Verification items for the finished model (mm, model axes). Face numbers are marked on the shaded views. A direction names the side the tool comes from. Round coordinates to 2 decimals unless told otherwise and drop trailing zeros. Order: outer loops, then holes, each group sorted by start corner. A loop starts at its lowest first (then second) coordinate and runs counter-clockwise, first axis right, second up. Notation, with made-up numbers: (67.5, 0) -> (97.5, 0) arc R11 ccw to (97.5, 4) -> close; hole circle Ø8 at (-30.75, 21.5). An arc over 180 degrees is marked (long way). Return JSON: item names as keys, results as strings. Group by question number.
Item 1: Depth check by flat-ended pin: pin 1 Ø2 at (y, z) = (-27, 3.5) entering from -X; pin 2 Ø1.6 at (x, z) = (-4.5, 3) entering from +Y; pin 3 Ø5 at (x, y) = (6, -23.5) entering from +Z. Enter the tip coordinate at first touch or a pass-through.
Item 2: Scan lines: probe 1 along X at (y, z) = (-23, 0.7); probe 2 along Z at (x, y) = (1.5, -26.5); probe 3 along X at (y, z) = (-24.75, 2.25). Record each from-to range of solid material in increasing order. Write a range as from..to.
Item 3: Sectioned sample at D-D on x = 7.5. Record the cut outline in (y, z).
Item 4: Sectioned sample at C-C on z = 2.5. Record the cut outline in (x, y).
Item 5: Access from +Z, -Z, +X, -X, +Y, -Y to the whole of each face (thin tool, end or side, straight path). Record for the marked faces 1, 2 and 3.
Item 6: Sectioned sample at A-A on y = -26. Record the cut outline in (x, z), plus the area to 3 significant figures.
Item 7: Sectioned sample at B-B on x = -4.25. Record the cut outline in (y, z), plus the area to 3 significant figures.
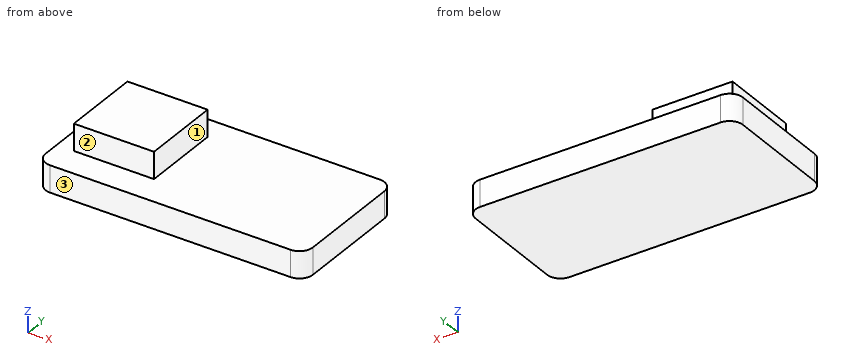
```python
from build123d import *

# Parameters (mm, degrees)
SKETCH1_W           = 20
SKETCH1_H           = 10
BOSS_EXTRUDE1_DEPTH = 2
FILLET1_R           = 1
SKETCH2_W           = 6
SKETCH2_H           = 6
BOSS_EXTRUDE2_DEPTH = 2


with BuildPart() as part:
    # Sketch1 → Boss-Extrude1 (new body)
    with BuildSketch(Plane.XY):
        with Locations((0, -27.096458497)):
            Rectangle(SKETCH1_W, SKETCH1_H)
    extrude(amount=BOSS_EXTRUDE1_DEPTH)

    # Fillet1
    fillet1_edges = [part.edges().sort_by_distance(p)[0] for p in [
        (-10, -22.096458497, 1),
        (10, -22.096458497, 1),
        (10, -32.096458497, 1),
        (-10, -32.096458497, 1),
    ]]
    fillet(fillet1_edges, radius=FILLET1_R)

    # Sketch2 → Boss-Extrude2 (add)
    with BuildSketch(Plane.XY.offset(2)):
        with Locations((-5.714480975, -26.862957006)):
            Rectangle(SKETCH2_W, SKETCH2_H)
    extrude(amount=BOSS_EXTRUDE2_DEPTH)


solid = part.part
```
Recorded:
{
 "1": {"pin 1": "x = -8.71", "pin 2": "y = -23.86", "pin 3": "z = 2"},
 "2": {"probe 1": "-10..10", "probe 2": "0..2", "probe 3": "-8.71..-2.71"},
 "3": {"outline": "(-32.1, 0) -> (-22.1, 0) -> (-22.1, 2) -> (-32.1, 2) -> close"},
 "4": {"outline": "(-8.71, -29.86) -> (-2.71, -29.86) -> (-2.71, -23.86) -> (-8.71, -23.86) -> close"},
 "5": {"face 1": "+Z, +X, +Y, -Y", "face 2": "+Z, +X, -X, -Y", "face 3": "+Z, -Z, +X, -X, -Y"},
 "6": {"outline": "(-10, 0) -> (10, 0) -> (10, 2) -> (-2.71, 2) -> (-2.71, 4) -> (-8.71, 4) -> (-8.71, 2) -> (-10, 2) -> close", "area": "52.0 mm²"},
 "7": {"outline": "(-32.1, 0) -> (-22.1, 0) -> (-22.1, 2) -> (-23.86, 2) -> (-23.86, 4) -> (-29.86, 4) -> (-29.86, 2) -> (-32.1, 2) -> close", "area": "32.0 mm²"}
}
